from build123d import *

# Parameters (mm, degrees)
PAD_DEPTH       = 15
SKETCH001_R     = 2.8
POCKET_DEPTH    = 8.2
SKETCH002_W     = 20
SKETCH002_H     = 15
PAD001_DEPTH    = 30
POCKET001_DEPTH = 15.001
SKETCH004_R     = 2.2
HOLE_DEPTH      = 23.678107
HOLE_TIPS_R     = 2.2
SKETCH005_W     = 2.5
SKETCH005_H     = 12
POCKET002_DEPTH = 15.001


with BuildPart() as part:
    # Sketch → Pad (new body)
    with BuildSketch(Plane.XY):
        Polygon((-30.5, -31), (-30.5, 0), (30.5, 0), (30.5, -31), (20.5, -31), (20.5, -10), (-20.5, -10), (-20.5, -31), align=None)
    extrude(amount=PAD_DEPTH)

    # Sketch001 (on Face10 of Pad) → Pocket (cut)
    with BuildSketch(Plane.XY.offset(15)):
        with Locations((-25, -15.5)):
            Circle(SKETCH001_R)
        with Locations((-25, -25.5)):
            Circle(SKETCH001_R)
        with Locations((25, -15.5)):
            Circle(SKETCH001_R)
        with Locations((25, -25.5)):
            Circle(SKETCH001_R)
    extrude(amount=-POCKET_DEPTH, mode=Mode.SUBTRACT)

    # Sketch002 (on Face3 of Pocket) → Pad001 (join)
    with BuildSketch(Plane(origin=(0, 0, 0), x_dir=(-1, 0, 0), z_dir=(0, 1, 0))):
        with Locations((0, 7.5)):
            Rectangle(SKETCH002_W, SKETCH002_H)
    extrude(amount=PAD001_DEPTH)

    # Sketch003 (on Face14 of Pad001) → Pocket001 (cut, through all)
    with BuildSketch(Plane.XY.offset(15)):
        with BuildLine():
            ThreePointArc((-1.25, 18.276743), (0, 5.6), (1.25, 18.276743))
            Line((1.25, 30), (1.25, 18.276743))
            Line((1.25, 30), (-1.25, 30))
            Line((-1.25, 18.276743), (-1.25, 30))
        make_face()
    extrude(amount=-POCKET001_DEPTH, mode=Mode.SUBTRACT)

    # Sketch004 (on Face24 of Pocket001) → Hole (cut)
    with BuildSketch(Plane.YZ.offset(10)):
        with Locations((24, 7.5)):
            Circle(SKETCH004_R)
    extrude(amount=-HOLE_DEPTH, mode=Mode.SUBTRACT)

    # Hole tips → Hole tip 1 section 0
    with BuildSketch(Plane.YZ.offset(-13.678107), mode=Mode.PRIVATE) as hole_tip_1_s0:
        with Locations((24, 7.5)):
            Circle(HOLE_TIPS_R)
    loft([hole_tip_1_s0.sketch, Vertex(-15, 24, 7.5)], mode=Mode.SUBTRACT)

    # Sketch005 (on Face14 of Hole) → Pocket002 (cut, through all)
    with BuildSketch(Plane.XY.offset(15)):
        with Locations((-8.75, 24)):
            Rectangle(SKETCH005_W, SKETCH005_H)
        with Locations((8.75, 24)):
            Rectangle(SKETCH005_W, SKETCH005_H)
    extrude(amount=-POCKET002_DEPTH, mode=Mode.SUBTRACT)


solid = part.part
Design review of the part built by this model. Coordinates are the model's own, in mm. A direction names the side the tool comes from. Coordinates: 2 decimals unless noted, no trailing zeros. Loops run counter-clockwise (first coordinate to the right, second up) from the corner with the lowest first, then second, coordinate; pieces in that order, holes last. Notation, with made-up numbers: (6.5, 6) -> (19.5, 6) arc R32 ccw to (19.5, 36) -> close; hole circle Ø7 at (27.5, 61.25). An arc over 180 degrees is marked (long way). Use a Markdown table: item, result. Add a question column.
Item 1: We need section A-A, the plane z = 12.5. Write out the cut boundary in (x, y), and give its area (3 significant figures).
Item 2: We need section D-D, the plane x = -25. Write out the cut boundary in (y, z).
Item 3: We need section B-B, the plane y = -25.5. Write out the cut boundary in (x, z).
Item 4: We need section C-C, the plane z = 3.5. Write out the cut boundary in (x, y), and give its area (3 significant figures).
Item 5: Wall thickness on L1, parallel to Y at x = -25, z = 11.5; L2, parallel to X at y = -24, z = 6.25; L3, parallel to X at y = 12, z = 5.5: over which ranges is each line inside the solid? List them lowest first. Write a range as from..to.
Item 6: The part is to be moulded in two halves that separate along X. For faces 6 (the flat face through (-25, -15, 6.8)), 7 (the flat face through (25, -15, 6.8)), 8 (the flat face through (9, 18, 8)), 9 (the flat face through (10, 9, 7)), say which applies: +X half, -X half, draft (parallel to the pull), parting line (faces both ways), or undercut.
Item 7: Clearance check with flat-ended pins moving along their axes: P1, Ø3, axis at x = -6.5, z = 8, coming from the -Y side; P2, Ø5, axis at y = 24, z = 7.5, coming from the -X side; P3, Ø0.8, axis at x = -8.5, z = 11, coming from the +Y side; P4, Ø1, axis at x = -12, y = 4, coming from the +Z side. State where each tip first meets the part, or that it passes through.
Item 8: Machinability: for faces 1 (the flat face through (-1.25, 27, 8)), 2 (the flat face through (-7.5, 21, 8)), 3 (the flat face through (-25, -25, 6.8)), 4 (the flat face through (0, -10, 7)), 5 (the flat face through (20, 0, 7)), which of the approach directions +Z, -Z, +X, -X, +Y, -Y give a long, thin tool a straight path to every point of the face, cutting with its end or side? Answer none if there is none.
Numbers:
| question | item | result |
|---|---|---|
| 1 | outline | (-30.5, -31) -> (-20.5, -31) -> (-20.5, -10) -> (20.5, -10) -> (20.5, -31) -> (30.5, -31) -> (30.5, 0) -> (10, 0) -> (10, 18) -> (7.5, 18) -> (7.5, 30) -> (1.25, 30) -> (1.25, 18.28) arc R6.4 cw (long way) to (-1.25, 18.28) -> (-1.25, 30) -> (-7.5, 30) -> (-7.5, 18) -> (-10, 18) -> (-10, 0) -> (-30.5, 0) -> close; hole circle Ø5.6 at (-25, -25.5); hole circle Ø5.6 at (-25, -15.5); hole circle Ø5.6 at (25, -25.5); hole circle Ø5.6 at (25, -15.5) |
| 1 | area | 1,310 mm^2 |
| 2 | outline | (-31, 0) -> (0, 0) -> (0, 15) -> (-12.7, 15) -> (-12.7, 6.8) -> (-18.3, 6.8) -> (-18.3, 15) -> (-22.7, 15) -> (-22.7, 6.8) -> (-28.3, 6.8) -> (-28.3, 15) -> (-31, 15) -> close |
| 3 | outline | (-30.5, 0) -> (-20.5, 0) -> (-20.5, 15) -> (-22.2, 15) -> (-22.2, 6.8) -> (-27.8, 6.8) -> (-27.8, 15) -> (-30.5, 15) -> close; (20.5, 0) -> (30.5, 0) -> (30.5, 15) -> (27.8, 15) -> (27.8, 6.8) -> (22.2, 6.8) -> (22.2, 15) -> (20.5, 15) -> close |
| 4 | outline | (-30.5, -31) -> (-20.5, -31) -> (-20.5, -10) -> (20.5, -10) -> (20.5, -31) -> (30.5, -31) -> (30.5, 0) -> (10, 0) -> (10, 18) -> (7.5, 18) -> (7.5, 30) -> (1.25, 30) -> (1.25, 18.28) arc R6.4 cw (long way) to (-1.25, 18.28) -> (-1.25, 30) -> (-7.5, 30) -> (-7.5, 18) -> (-10, 18) -> (-10, 0) -> (-30.5, 0) -> close |
| 4 | area | 1,410 mm^2 |
| 5 | L1 | y = -31..-28.3, -22.7..-18.3, -12.7..0 |
| 5 | L2 | x = -30.5..-20.5, 20.5..30.5 |
| 5 | L3 | x = -10..-6.4, 6.4..10 |
| 6 | face 6 | undercut |
| 6 | face 7 | undercut |
| 6 | face 8 | draft |
| 6 | face 9 | +X half |
| 7 | P1 | stops at y = -10 |
| 7 | P2 | stops at x = -7.5 |
| 7 | P3 | stops at y = 18 |
| 7 | P4 | passes through |
| 8 | face 1 | +Z, -Z, +Y |
| 8 | face 2 | +Z, -Z, -X, +Y |
| 8 | face 3 | +Z |
| 8 | face 4 | +Z, -Z, -Y |
| 8 | face 5 | +Z, -Z, +X, +Y |
